from build123d import *

# Parameters (mm, degrees)
SKETCH1_R                         = 5
BOSS_EXTRUDE3_DEPTH               = 2
SKETCH5_W                         = 2
SKETCH5_H                         = 11
BOSS_EXTRUDE4_DEPTH               = 197.88316
SKETCH6_R                         = 2.5
BOSS_EXTRUDE5_DEPTH               = 2
SKETCH8_W                         = 2
SKETCH8_H                         = 11
BOSS_EXTRUDE6_DEPTH               = 4
CUT_EXTRUDE8_REACH                = 209.363
SKETCH10_R                        = 2
SKETCH11_R                        = 4
SKETCH11_R_2                      = 2.5
BOSS_EXTRUDE7_DEPTH               = 4
CUT_EXTRUDE9_REACH                = 209.363
SKETCH12_R                        = 2.5
FILLET1_R                         = 1
M3_5X0_6_TAPPED_HOLE7_D           = 2.9
M3_5X0_6_TAPPED_HOLE7_DEPTH       = 2
M3_5X0_6_TAPPED_HOLE7_CSINK_D     = 3.55
M3_5X0_6_TAPPED_HOLE7_CSINK_ANGLE = 90


with BuildPart() as part:
    # Sketch1 → Boss-Extrude3 (new body)
    with BuildSketch(Plane(origin=(0, 0, 0), x_dir=(1, 0, 0), z_dir=(0, 1, 0))):
        with BuildLine():
            Line((-206.5, 4), (-8.61684397, 4))
            ThreePointArc((-8.61684397, 4), (9.5, 0), (-8.61684397, -4))
            Line((-8.61684397, -4), (-206.5, -4))
            Line((-206.5, -4), (-206.5, 4))
        make_face()
        with Locations(Location((0, 0, 0), (0, 0, 270))):
            Circle(SKETCH1_R, mode=Mode.SUBTRACT)
    extrude(amount=BOSS_EXTRUDE3_DEPTH)

    # Sketch5 → Boss-Extrude4 (add)
    with BuildSketch(Plane.ZY.offset(206.5)):
        with Locations((3, 7.5)):
            Rectangle(SKETCH5_W, SKETCH5_H)
    extrude(amount=-BOSS_EXTRUDE4_DEPTH)


with BuildPart() as boss_extrude5_tool:
    # Sketch6 → Boss-Extrude5 (new body)
    with BuildSketch(Plane(origin=(0, 13, 0), x_dir=(1, 0, 0), z_dir=(0, 1, 0))):
        with BuildLine():
            Line((-206.5, 4), (-8.61684397, 4))
            ThreePointArc((-8.61684397, 4), (9.5, 0), (-8.61684397, -4))
            Line((-8.61684397, -4), (-206.5, -4))
            Line((-206.5, -4), (-206.5, 4))
        make_face()
        with Locations(Location((0, 0, 0), (0, 0, 270))):
            Circle(SKETCH6_R, mode=Mode.SUBTRACT)
    extrude(amount=BOSS_EXTRUDE5_DEPTH)


with BuildPart() as part_1:
    add(part.part)


with BuildPart() as part_2:
    # Boss-Extrude5: joined with boss_extrude5_tool
    add(part_1.part.fuse(boss_extrude5_tool.part, tol=0.00001))

    # Sketch8 → Boss-Extrude6 (add)
    with BuildSketch(Plane(origin=(-8.61684397, 0, 0), x_dir=(0, 0, -1), z_dir=(1, 0, 0))):
        with Locations((-3, 7.5)):
            Rectangle(SKETCH8_W, SKETCH8_H)
    extrude(amount=BOSS_EXTRUDE6_DEPTH)

    # Sketch10 → Cut-Extrude8 (cut, up to next)
    with BuildSketch(Plane(origin=(0, 0, 2), x_dir=(-1, 0, 0), z_dir=(0, 0, -1)), mode=Mode.PRIVATE) as cut_extrude8_sk1:
        with Locations((201.5, 7.5)):
            Circle(SKETCH10_R)
    cut_extrude8_tool1 = extrude(cut_extrude8_sk1.sketch, amount=-CUT_EXTRUDE8_REACH, mode=Mode.PRIVATE) & part_2.part
    # Sketch10 → Cut-Extrude8 (cut, up to next)
    with BuildSketch(Plane(origin=(0, 0, 2), x_dir=(-1, 0, 0), z_dir=(0, 0, -1)), mode=Mode.PRIVATE) as cut_extrude8_sk2:
        with Locations((191.5, 7.5)):
            Circle(SKETCH10_R)
    cut_extrude8_tool2 = extrude(cut_extrude8_sk2.sketch, amount=-CUT_EXTRUDE8_REACH, mode=Mode.PRIVATE) & part_2.part
    add(cut_extrude8_tool1.solids().sort_by_distance((-201.5, 7.5, 2))[0], mode=Mode.SUBTRACT)
    add(cut_extrude8_tool2.solids().sort_by_distance((-191.5, 7.5, 2))[0], mode=Mode.SUBTRACT)

    # Sketch11 → Boss-Extrude7 (add)
    with BuildSketch(Plane(origin=(0, 0, 2), x_dir=(-1, 0, 0), z_dir=(0, 0, -1))):
        with Locations((11.5, 7.5)):
            Circle(SKETCH11_R)
        with Locations((11.5, 7.5)):
            Circle(SKETCH11_R_2, mode=Mode.SUBTRACT)
    extrude(amount=BOSS_EXTRUDE7_DEPTH)

    # Sketch12 → Cut-Extrude9 (cut, up to next)
    with BuildSketch(Plane(origin=(0, 0, 2), x_dir=(-1, 0, 0), z_dir=(0, 0, -1)), mode=Mode.PRIVATE) as cut_extrude9_sk1:
        with Locations((11.5, 7.5)):
            Circle(SKETCH12_R)
    cut_extrude9_tool1 = extrude(cut_extrude9_sk1.sketch, amount=-CUT_EXTRUDE9_REACH, mode=Mode.PRIVATE) & part_2.part
    add(cut_extrude9_tool1.solids().sort_by_distance((-11.5, 7.5, 2))[0], mode=Mode.SUBTRACT)

    # Fillet1
    fillet1_edges = [part_2.edges().sort_by_distance(p)[0] for p in [
        (-7.5, 7.5, 2),
    ]]
    fillet(fillet1_edges, radius=FILLET1_R)

    # M3.5x0.6 Tapped Hole7
    with Locations(Plane(origin=(0, 15, 0), x_dir=(1, 0, 0), z_dir=(0, 1, 0))):
        with Locations((-176, 0), (-192, 0)):
            CounterSinkHole(M3_5X0_6_TAPPED_HOLE7_D / 2, M3_5X0_6_TAPPED_HOLE7_CSINK_D / 2, depth=M3_5X0_6_TAPPED_HOLE7_DEPTH, counter_sink_angle=M3_5X0_6_TAPPED_HOLE7_CSINK_ANGLE)


solid = part_2.part
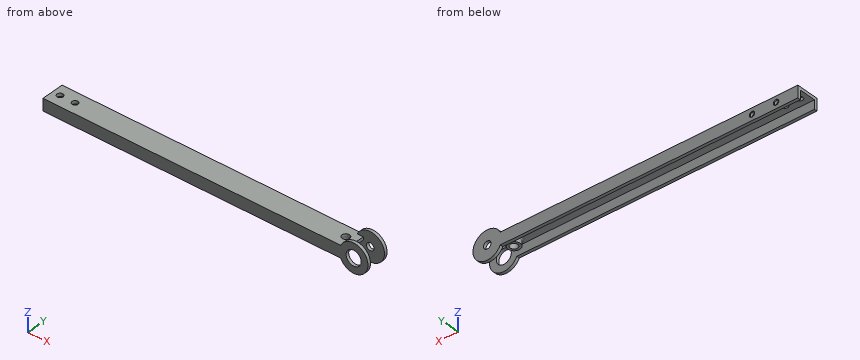
The listing builds one solid part. Answer for the finished solid, in the listing's coordinates (mm). Round coordinates to 2 decimals unless told otherwise and drop trailing zeros. Write each loop counter-clockwise with the first axis right and the second up, starting at its lowest first coordinate (ties: lowest second). Pieces come first, ordered by that corner, then holes. Notation, with made-up numbers: M 82,-12 L 121,-12 A21 cw 121,-1 Z; hole C -14.5,-1 d4. An arc over 180 degrees is marked long. Write each question's results on one line, items separated by ' | '. Start each with the question number.
Item 1: A cutting plane is placed at C-C on z = 7. Write down the section's boundary in (x, y).
Item 2: Flat-ended cylindrical pins translate along their axes: pin 1 Ø3 at (y, z) = (2, -7) entering from +X; pin 2 Ø1 at (x, y) = (-97, 13.5) entering from -Z; pin 3 Ø6 at (x, y) = (-11.5, 7.5) entering from +Z; pin 4 Ø2.5 at (x, y) = (-11, 8) entering from -Z. Find the tip coordinate at first contact, or state that the pin passes through.
Item 3: A cutting plane is placed at A-A on x = 0. Write down the section's boundary in (y, z).
Item 4: Straight lines are drawn through the part: L1, parallel to Y at x = -11.5, z = 2.7; L2, parallel to Z at x = -192, y = 13.5; L3, parallel to Y at x = -31, z = 1.75. For each, find the intervals that lie inside material, in ascending order. Write a range as [from, to].
Item 5: A cutting plane is placed at B-B on x = -31. Write down the section's boundary in (y, z).
Check sheet entries:
1) outline: M -6.42,0 L 6.42,0 L 6.42,2 L -6.42,2 Z; M -6.42,13 L 6.42,13 L 6.42,15 L -6.42,15 Z
2) pin 1: x = 7.75 | pin 2: z = -4 | pin 3: z = 4 | pin 4: through
3) outline: M 0,-9.5 L 2,-9.5 L 2,-5 L 0,-5 Z; M 0,5 L 2,5 L 2,9.5 L 0,9.5 Z; M 13,-9.5 L 15,-9.5 L 15,-2.5 L 13,-2.5 Z; M 13,2.5 L 15,2.5 L 15,9.5 L 13,9.5 Z
4) L1: [0, 5], [10, 15] | L2: [-4, -1.45], [1.45, 4] | L3: [0, 2], [13, 15]
5) outline: M 0,-4 L 2,-4 L 2,2 L 13,2 L 13,-4 L 15,-4 L 15,4 L 0,4 Z
